```python
from build123d import *

# Parameters (mm, degrees)
SKETCH1_R           = 6
BOSS_EXTRUDE1_DEPTH = 3
SKETCH3_R           = 4
BOSS_EXTRUDE2_DEPTH = 25
FILLET1_R           = 1
CHAMFER1_SIZE       = 0.5


with BuildPart() as part:
    # Sketch1 → Boss-Extrude1 (new body)
    with BuildSketch(Plane(origin=(0, 0, 0), x_dir=(0, 0, -1), z_dir=(1, 0, 0))):
        Circle(SKETCH1_R)
    extrude(amount=BOSS_EXTRUDE1_DEPTH)

    # Sketch3 → Boss-Extrude2 (add)
    with BuildSketch(Plane.ZY):
        Circle(SKETCH3_R)
    extrude(amount=BOSS_EXTRUDE2_DEPTH)

    # Fillet1
    fillet1_edges = [part.edges().sort_by_distance(p)[0] for p in [
        (3, 0, 6),
    ]]
    fillet(fillet1_edges, radius=FILLET1_R)

    # Chamfer1
    chamfer1_edges = [part.edges().sort_by_distance(p)[0] for p in [
        (-25, 0, -4),
    ]]
    chamfer(chamfer1_edges, length=CHAMFER1_SIZE)


solid = part.part
```
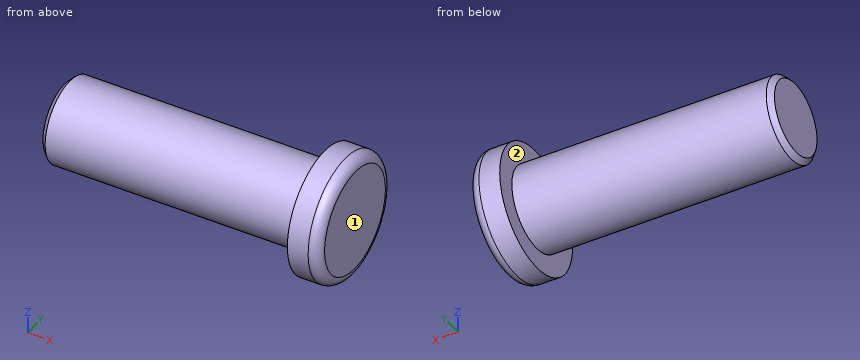
Here's how the part is built. I have some questions about the finished solid (model axes, mm). Face numbers are marked on the shaded views. A direction names the side the tool comes from. Give positions to 0.01 mm unless a question says otherwise; leave off trailing zeros. Loops run counter-clockwise (first coordinate to the right, second up) from the corner with the lowest first, then second, coordinate; pieces in that order, holes last. Notation, with made-up numbers: (53.5, -39.75) -> (88.5, -39.75) arc R37 ccw to (88.5, -1.75) -> close; hole circle Ø4 at (13, 75). An arc over 180 degrees is marked (long way). Use one line per item in the form item = value. Start each with the question number.
1) Imagine slicing it at C-C (x = -4.25). Please give me the cut outline in (y, z), then the cut area to 3 significant figures.
2) Which directions (+Z, -Z, +X, -X, +Y, -Y) give clear straight access to the entire face, cutting with the end or side of a thin tool? Please do the marked faces 1 and 2.
3) Imagine slicing it at A-A (y = 0). Please give me the cut outline in (x, z).
4) For P1, Ø3, axis at y = 4.5, z = -2, coming from the -X side; P2, Ø6, axis at x = -18.5, z = 2, coming from the -Y side; P3, Ø3, axis at x = -3.5, z = 4, coming from the +Y side; P4, Ø4, axis at x = -19.5, y = -1, coming from the -Z side, each with a flat end and sliding along its axis, tell me the tip position at first contact or that it passes through.
5) Please list where these lines run through material, in increasing order: line 1 along X through (y, z) = (0.75, -4.5); line 2 along Z through (x, y) = (-11, -0.75); line 3 along Y through (x, z) = (-10.5, -0.5).
Check values:
q1.outline = circle Ø8 at (0, 0)
q1.area = 50.3 mm^2
q2.face_1 = +Z, -Z, +X, +Y, -Y
q2.face_2 = -X
q3.outline = (-25, -3.5) -> (-24.5, -4) -> (0, -4) -> (0, -6) -> (2, -6) arc R1 ccw to (3, -5) -> (3, 5) arc R1 ccw to (2, 6) -> (0, 6) -> (0, 4) -> (-24.5, 4) -> (-25, 3.5) -> close
q4.P1 = -25
q4.P2 = -4
q4.P3 = 3.12
q4.P4 = -4
q5.line_1 = 0 to 3
q5.line_2 = -3.93 to 3.93
q5.line_3 = -3.97 to 3.97
